```python
from build123d import *

# Parameters (mm, degrees)
SKETCH_1_R               = 14.5
EXTRUDE_1_DEPTH          = 41.7
CHAMFER_1_SIZE           = 10.5
SKETCH_2_R               = 2
CUT_EXTRUDE_1_DEPTH      = 47.469237136
CHAMFER_2_SIZE           = 5
CHAMFER_2_SIZE2          = 1
SKETCH_3_W               = 2
SKETCH_3_H               = 1.5
CUT_EXTRUDE_2_DEPTH      = 47.469237136
CUT_EXTRUDE_2_DEPTH_BACK = 47.469237136
SKETCH_5_W               = 6.979253001
SKETCH_5_H               = 12
SKETCH_6_R               = 8.65
CUT_EXTRUDE_3_DEPTH      = 5.6
CHAMFER_3_SIZE           = 0.5
SKETCH_7_R               = 8.15
CUT_EXTRUDE_4_DEPTH      = 15.6
CHAMFER_4_SIZE           = 0.5
SKETCH_8_R               = 7
CUT_EXTRUDE_5_DEPTH      = 17.5
CUT_EXTRUDE_6_DEPTH      = 8
CUT_EXTRUDE_7_DEPTH      = 8
SKETCH_10_R              = 1.5
CUT_EXTRUDE_8_DEPTH      = 7


with BuildPart() as part:
    # 草图1 → 凸台-拉伸1 (new body)
    with BuildSketch(Plane(origin=(0, 0, 0), x_dir=(1, 0, 0), z_dir=(0, 1, 0))):
        with Locations(Location((0, 0, 0), (0, 0, 270))):
            Circle(SKETCH_1_R)
    extrude(amount=EXTRUDE_1_DEPTH)

    # 倒角1
    chamfer_1_edges = [part.edges().sort_by_distance(p)[0] for p in [
        (0, 41.7, -14.5),
    ]]
    chamfer(chamfer_1_edges, length=CHAMFER_1_SIZE)

    # 草图2 → 切除-拉伸1 (cut, through all)
    with BuildSketch(Plane(origin=(0, 41.7, 0), x_dir=(1, 0, 0), z_dir=(0, 1, 0))):
        with Locations(Location((0, 0, 0), (0, 0, 270))):
            Circle(SKETCH_2_R)
    extrude(amount=-CUT_EXTRUDE_1_DEPTH, mode=Mode.SUBTRACT)

    # 倒角2
    chamfer_2_edges = [part.edges().sort_by_distance(p)[0] for p in [
        (0, 0, -14.5),
    ]]
    chamfer_2_side = [part.faces().sort_by_distance(p)[0] for p in [
        (0, 0, -14.089878067),
    ]]
    chamfer(chamfer_2_edges, length=CHAMFER_2_SIZE, length2=CHAMFER_2_SIZE2, reference=chamfer_2_side[0])

    # 草图3 → 切除-旋转1 (revolve, cut)
    with BuildSketch(Plane.XY, mode=Mode.PRIVATE) as cut_revolve_1_sk:
        with Locations((13.5, 4.25)):
            Rectangle(SKETCH_3_W, SKETCH_3_H)
        with Locations((13.5, 8.25)):
            Rectangle(SKETCH_3_W, SKETCH_3_H)
        with Locations((13.5, 12.25)):
            Rectangle(SKETCH_3_W, SKETCH_3_H)
    revolve(cut_revolve_1_sk.sketch.rotate(Axis((0, 0, 0), (0, 1, 0)), 90), axis=Axis((0, 0, 0), (0, 1, 0)), mode=Mode.SUBTRACT)

    # 草图5 → 切除-拉伸2 (cut, two sides: drawn at the far end of the back side and taken through both)
    with BuildSketch(Plane.XY.offset(-CUT_EXTRUDE_2_DEPTH_BACK)):
        with Locations((14.389626501, 20.5)):
            Rectangle(SKETCH_5_W, SKETCH_5_H)
    extrude(amount=CUT_EXTRUDE_2_DEPTH + CUT_EXTRUDE_2_DEPTH_BACK, mode=Mode.SUBTRACT)

    # 草图6 → 切除-拉伸3 (cut)
    with BuildSketch(Plane.XZ):
        with Locations(Location((0, 0, 0), (0, 0, 270))):
            Circle(SKETCH_6_R)
    extrude(amount=-CUT_EXTRUDE_3_DEPTH, mode=Mode.SUBTRACT)

    # 倒角3
    chamfer_3_edges = [part.edges().sort_by_distance(p)[0] for p in [
        (0, 0, 8.65),
    ]]
    chamfer(chamfer_3_edges, length=CHAMFER_3_SIZE)

    # 草图7 → 切除-拉伸4 (cut)
    with BuildSketch(Plane.XZ):
        with Locations(Location((0, 0, 0), (0, 0, 270))):
            Circle(SKETCH_7_R)
    extrude(amount=-CUT_EXTRUDE_4_DEPTH, mode=Mode.SUBTRACT)

    # 倒角4
    chamfer_4_edges = [part.edges().sort_by_distance(p)[0] for p in [
        (0, 5.6, 8.15),
    ]]
    chamfer(chamfer_4_edges, length=CHAMFER_4_SIZE - 0.0001)  # a hair under: the kernel refuses the full size

    # 草图8 → 切除-拉伸5 (cut)
    with BuildSketch(Plane.XZ):
        with Locations(Location((0, 0, 0), (0, 0, 270))):
            Circle(SKETCH_8_R)
    extrude(amount=-CUT_EXTRUDE_5_DEPTH, mode=Mode.SUBTRACT)

    # 草图9 → 切除-拉伸6 (cut)
    with BuildSketch(Plane(origin=(10.9, 0, 0), x_dir=(0, 0, -1), z_dir=(1, 0, 0))):
        with BuildLine():
            ThreePointArc((-3.5, 20.5), (-5, 22), (-6.5, 20.5))
            Line((-6.5, 20.5), (-3.5, 20.5))
        make_face()
        with BuildLine():
            Line((-3.5, 20.5), (-6.5, 20.5))
            ThreePointArc((-6.5, 20.5), (-5, 19), (-3.5, 20.5))
        make_face()
        with BuildLine():
            ThreePointArc((6.5, 20.5), (5, 22), (3.5, 20.5))
            Line((3.5, 20.5), (6.5, 20.5))
        make_face()
        with BuildLine():
            Line((6.5, 20.5), (3.5, 20.5))
            ThreePointArc((3.5, 20.5), (5, 19), (6.5, 20.5))
        make_face()
    extrude(amount=-CUT_EXTRUDE_6_DEPTH, mode=Mode.SUBTRACT)

    # 草图9<3> → 切除-拉伸7 (cut)
    with BuildSketch(Plane(origin=(10.9, 0, 0), x_dir=(0, 0, -1), z_dir=(1, 0, 0))):
        with BuildLine():
            ThreePointArc((1.5, 20.5), (0, 22), (-1.5, 20.5))
            Line((-1.5, 20.5), (1.5, 20.5))
        make_face()
        with BuildLine():
            Line((1.5, 20.5), (-1.5, 20.5))
            ThreePointArc((-1.5, 20.5), (0, 19), (1.5, 20.5))
        make_face()
    extrude(amount=-CUT_EXTRUDE_7_DEPTH, mode=Mode.SUBTRACT)

    # 草图10 → 切除-拉伸8 (cut)
    with BuildSketch(Plane.XZ.offset(-17.5)):
        with Locations(Location((4.5, 0, 0), (0, 0, 270))):
            Circle(SKETCH_10_R)
    extrude(amount=-CUT_EXTRUDE_8_DEPTH, mode=Mode.SUBTRACT)


solid = part.part
```
Can you work these out from the model? Positions are in its coordinate system, mm. A direction names the side the tool comes from. Give positions to 0.01 mm unless a question says otherwise; leave off trailing zeros. Loops run counter-clockwise (first coordinate to the right, second up) from the corner with the lowest first, then second, coordinate; pieces in that order, holes last. Notation, with made-up numbers: M 73,43 L 78,43 A14 cw 78,62 Z; hole C -5,13.25 d8. An arc over 180 degrees is marked long. One line per item, written item: value.
(1) Suppose I cut it at C-C on x = 5.5. Count the separate pieces of the cut face and the enclosed holes in it, plus the area to 3 significant figures.
Returned:
separate pieces: 1
enclosed holes: 2
area: 714 mm^2
(2) I need wall thicknesses on line 1 (X direction, y = 16.65, z = 0); line 2 (Y direction, x = 12.75, z = -1.5); line 3 (Z direction, x = 9.5, y = 20.5). Which ranges of each line are inside material? Lowest first, please.
Returned:
line 1: -14.5 to -7, 7 to 10.9
line 2: 0.67 to 3.5, 5 to 7.5, 9 to 11.5, 13 to 14.5, 26.5 to 32.86
line 3: -10.95 to -6.5, -3.5 to -1.5, 1.5 to 3.5, 6.5 to 10.95
(3) Which directions (+Z, -Z, +X, -X, +Y, -Y) give clear straight access to the entire face, cutting with the end or side of a thin tool? Please do faces 1 (the face through (4.57, 22.92, 1.5)), 2 (the face through (12, 14.5, 0)), 3 (the face through (-3.755, 4.26, -11.923)), 4 (the face through (7, 19, -5)).
Returned:
face 1: -Y
face 2: +Z, -Z, +X
face 3: none
face 4: +X
(4) We'd pull the mould along Y, two halves only. Please class faces 5 (the face through (-9.579, 0.063, -2.127)), 6 (the face through (2.6, 3.01, -8.25)), 7 (the face through (-7, 9, -11)): released by +Y, released by -Y, zero draft, split by the parting line, or undercut.
Returned:
face 5: released by -Y
face 6: zero draft
face 7: undercut
(5) Suppose I cut it at B-B on y = 8.5. List the corners of the cut face in (x, z) for me, plus the area to 3 significant figures.
Returned:
outline: C 0,0 d25; hole C 0,0 d16.3
area: 282 mm^2
(6) Will these pins go through, and if not, where does the flat tip stop? pin 1 (0.9 mm diameter, centred on y = 21, z = -5, fed in from +X); pin 2 (10 mm diameter, centred on x = 0.5, z = -4, fed in from -Y); pin 3 (16 mm diameter, centred on x = 0, z = 0, fed in from -Y); pin 4 (13 mm diameter, centred on y = 23.5, z = -4, fed in from +X).
Returned:
pin 1: x = 2.9
pin 2: y = 0.12
pin 3: y = 15.6
pin 4: x = 14.5
(7) Suppose I cut it at A-A on y = 23. List the corners of the cut face in (x, z) for me, plus the area to 3 significant figures.
Returned:
outline: M 10.9,-9.56 L 10.9,9.56 A14.5 ccw long Z; hole C 0,0 d4; hole C 4.5,0 d3
area: 594 mm^2
